Work out the finished part from the listing and answer in its coordinate system (mm). A direction names the side the tool comes from. Coordinates: 2 decimals unless noted, no trailing zeros. Write each loop counter-clockwise with the first axis right and the second up, starting at its lowest first coordinate (ties: lowest second). Pieces come first, ordered by that corner, then holes. Notation, with made-up numbers: (-40, 71.25) - (8, 71.25) arc R15 cw to (8, 75.25) - close; hole circle Ø8 at (82, 25). An arc over 180 degrees is marked (long way). Use one line per item in the form item = value. Start each with the question number.
Item 1: For faces 1 (the cylindrical face through (7.493, 0.33, 59.16)), 2 (the flat face through (1, -2, 125)), determine the directions among +Z, -Z, +X, -X, +Y, -Y from which every point of the face is accessible in a straight line to the end or side of a thin tool.
Item 2: Consider probe 1 along Y at (x, z) = (0.25, 83); probe 2 along Z at (x, y) = (-0.75, -2.25). Determine where each line is inside the solid, lowest interval first.
Item 3: A cutting plane is placed at A-A (x = 0). Write down the section's boundary in (y, z).
Item 4: A cutting plane is placed at C-C (z = 15.5). Write down the section's boundary in (x, y), then the cut area to 3 significant figures.
Item 5: Given pin 1 (5 mm diameter, centred on x = -0.5, y = 0, fed in from -Z); pin 2 (5 mm diameter, centred on x = 5, z = 39.5, fed in from +Y); pin 3 (3 mm diameter, centred on x = 3.5, z = 74, fed in from -Y); pin 4 (4 mm diameter, centred on y = -2.5, z = 65.5, fed in from -X), each flat-ended and moving along its own axis, determine where each tip first touches the part or whether it passes through.
Autodesk Inventor part; units mm, degrees
ref_plane "YZ Plane" through (0, 0, 0) normal (1, 0, 0) x (0, 1, 0)
ref_plane "XZ Plane" through (0, 0, 0) normal (0, 1, 0) x (-1, 0, 0)
ref_plane "XY Plane" through (0, 0, 0) normal (0, 0, 1) x (1, 0, 0)
sketch "Sketch2" plane through (0, 0, 0) normal (0, 0, 1) x (-1, 0, 0)
  circle A0 centre (0, 0) radius 7.5
  dimension "d0" = 15
extrude "Extrusion1" add sketch "Sketch2" along normal blind 125
sketch "Sketch3" plane through (0, 0, 125) normal (0, 0, 1) x (1, 0, 0)
  circle A0 centre (0, 0) radius 2
  dimension "d3" = 4
extrude "Extrusion2" add sketch "Sketch3" along normal blind 5
chamfer "Chamfer1" distance 5 angle 45 1 edges at (7.5, 0, 125)
properties part number "Marcador"
Answer:
q1.face_1 = +Z, -Z
q1.face_2 = +Z
q2.probe_1 = -7.5 to 7.5
q2.probe_2 = 0 to 125
q3.outline = (-7.5, 0) - (7.5, 0) - (7.5, 120) - (2.5, 125) - (2, 125) - (2, 130) - (-2, 130) - (-2, 125) - (-2.5, 125) - (-7.5, 120) - close
q4.outline = circle Ø15 at (0, 0)
q4.area = 177 mm²
q5.pin_1 = 0
q5.pin_2 = 7.07
q5.pin_3 = -7.23
q5.pin_4 = -7.48
